from build123d import *

# Parameters (mm, degrees)
EXTRUDE_1_DEPTH     = 496
CUT_EXTRUDE_1_DEPTH = 497.805797068
CUT_EXTRUDE_2_REACH = 498.806
SKETCH_3_R          = 1.75


with BuildPart() as part:
    # Эскиз1 → Бобышка-Вытянуть1 (new body)
    with BuildSketch(Plane(origin=(0, 0, 0), x_dir=(0, 0, -1), z_dir=(1, 0, 0))):
        Polygon((0, 0), (20, 0), (20, 1.5), (1.5, 1.5), (1.5, 20), (0, 20), align=None)
    extrude(amount=EXTRUDE_1_DEPTH)

    # Эскиз2 → Вырез-Вытянуть1 (cut, through all)
    with BuildSketch(Plane.XZ):
        Polygon((0, 0), (0, -20), (20, -20), align=None)
    cut_extrude_1 = extrude(amount=-CUT_EXTRUDE_1_DEPTH, mode=Mode.SUBTRACT)

    # Эскиз3 → Вырез-Вытянуть2 (cut, up to next)
    with BuildSketch(Plane.XY, mode=Mode.PRIVATE) as cut_extrude_2_sk1:
        with Locations((8.5, 10)):
            Circle(SKETCH_3_R)
    cut_extrude_2_tool1 = extrude(cut_extrude_2_sk1.sketch, amount=-CUT_EXTRUDE_2_REACH, mode=Mode.PRIVATE) & part.part
    cut_extrude_2 = cut_extrude_2_tool1.solids().sort_by_distance((8.5, 10, 0))[0]
    add(cut_extrude_2, mode=Mode.SUBTRACT)

    # Зеркальное отражение1: Вырез-Вытянуть1, Вырез-Вытянуть2 across plane
    add(cut_extrude_1.mirror(Plane(origin=(248, 0, 0), x_dir=(0, 0, 1), z_dir=(1, 0, 0))), mode=Mode.SUBTRACT)
    add(cut_extrude_2.mirror(Plane(origin=(248, 0, 0), x_dir=(0, 0, 1), z_dir=(1, 0, 0))), mode=Mode.SUBTRACT)


solid = part.part
Could you check a few things on this model? Use its own coordinates, in mm. A direction names the side the tool comes from. Give positions to 0.01 mm unless a question says otherwise; leave off trailing zeros. Order: outer loops, then holes, each group sorted by start corner. A loop starts at its lowest first (then second) coordinate and runs counter-clockwise, first axis right, second up.
1. For faces 1 (the flat face through (245, 10, 0)), 2 (the flat face through (245, 1.5, -11)), which set-ups out of +Z, -Z, +X, -X, +Y, -Y let a thin tool reach every point of the face, with its end or its side?
2. I need wall thicknesses on L1, parallel to Y at x = 8.5, z = -1.15; L2, parallel to Y at x = 70, z = -9.25; L3, parallel to Z at x = 287, y = 14.75. Which ranges of each line are inside material? Lowest first, please.
3. Suppose I cut it at A-A (x = 419). List the corners of the cut face in (y, z) for me, plus the area to 4 significant figures.
4. Suppose I cut it at B-B (z = -5.25). List the corners of the cut face in (x, y) for me, plus the area to 3 significant figures.
5. Will these pins go through, and if not, where does the flat tip stop? P1, Ø10, axis at x = 427.5, y = 13.5, coming from the -Z side; P2, Ø1.5, axis at x = 164.5, z = -9, coming from the +Y side.
Solved:
1. face 1: +Z, +X, -X, +Y, -Y
1. face 2: -Z, +X, -X, +Y
2. L1: y = 0 to 8.25, 11.75 to 20
2. L2: y = 0 to 1.5
2. L3: z = -1.5 to 0
3. outline: (0, -20) - (1.5, -20) - (1.5, -1.5) - (20, -1.5) - (20, 0) - (0, 0) - close
3. area: 57.75 mm2
4. outline: (5.25, 0) - (490.75, 0) - (490.75, 1.5) - (5.25, 1.5) - close
4. area: 728 mm2
5. P1: stops at z = -1.5
5. P2: stops at y = 1.5
